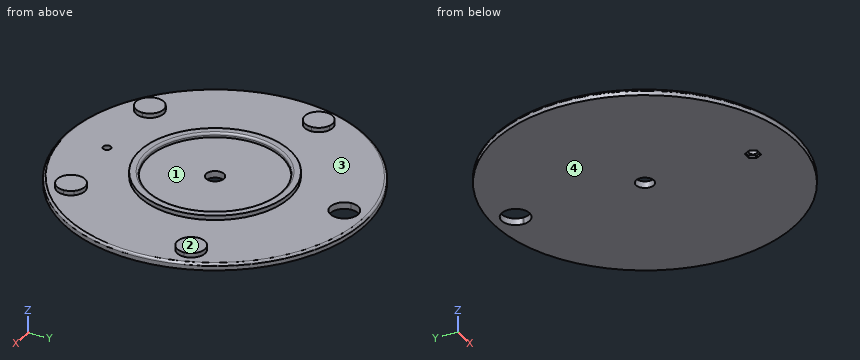
```python
from build123d import *

# Parameters (mm, degrees)
F0_R     = 67.5
F0_R_2   = 33.75
F1_DEPTH = 3
F0_R_3   = 30
F0_R_4   = 4
F2_DEPTH = 5
F3_START = 1
F0_R_5   = 1.75
F3_DEPTH = 2
F4_R     = 1


with BuildPart() as f1:
    # F0 (on Top) → F1 (new body)
    with BuildSketch(Plane.XY):
        Circle(F0_R)
        with BuildLine():
            ThreePointArc((-6.240649333, 56.8082458443), (-0.1709410263, 63.3976618959), (6.25, 57.15))
            ThreePointArc((6.25, 57.15), (6.2476618959, 56.9790589737), (6.240649333, 56.8082458443))
            ThreePointArc((6.240649333, 56.8082458443), (33.5919271685, 46.2353212285), (52.0993856897, 23.4899236005))
            ThreePointArc((52.0993856897, 23.4899236005), (57.8868692347, 22.8152624917), (60.6028799063, 17.6603212285))
            ThreePointArc((60.6028799063, 17.6603212285), (59.3068679409, 13.8497435095), (55.9563190893, 11.6195031725))
            ThreePointArc((55.9563190893, 11.6195031725), (56.8507965465, 5.8403280749), (57.15, 0))
            ThreePointArc((57.15, 0), (52.2635598843, -23.1223443496), (38.4398404822, -42.290674666))
            ThreePointArc((38.4398404822, -42.290674666), (39.480983044, -44.1421129506), (39.8419271685, -46.2353212285))
            ThreePointArc((39.8419271685, -46.2353212285), (35.3599862925, -52.2300244684), (28.3422577496, -49.6269979513))
            ThreePointArc((28.3422577496, -49.6269979513), (0, -57.15), (-28.3422577496, -49.6269979513))
            ThreePointArc((-28.3422577496, -49.6269979513), (-37.2655849953, -51.2916774434), (-38.4398404822, -42.290674666))
            ThreePointArc((-38.4398404822, -42.290674666), (-54.3528799063, -17.6603212285), (-55.9563190893, 11.6195031725))
            ThreePointArc((-55.9563190893, 11.6195031725), (-60.2969831331, 19.5916774434), (-52.0993856897, 23.4899236005))
            ThreePointArc((-52.0993856897, 23.4899236005), (-33.5919271685, 46.2353212285), (-6.240649333, 56.8082458443))
        make_face(mode=Mode.SUBTRACT)
        with BuildLine():
            ThreePointArc((6.240649333, 56.8082458443), (0, 50.9), (-6.240649333, 56.8082458443))
            ThreePointArc((-6.240649333, 56.8082458443), (-33.5919271685, 46.2353212285), (-52.0993856897, 23.4899236005))
            ThreePointArc((-52.0993856897, 23.4899236005), (-49.1979386431, 21.1943105569), (-48.1028799063, 17.6603212285))
            ThreePointArc((-48.1028799063, 17.6603212285), (-50.5423021872, 12.7063331939), (-55.9563190893, 11.6195031725))
            ThreePointArc((-55.9563190893, 11.6195031725), (-54.3528799063, -17.6603212285), (-38.4398404822, -42.290674666))
            ThreePointArc((-38.4398404822, -42.290674666), (-31.4987188906, -40.346265353), (-27.3419271685, -46.2353212285))
            ThreePointArc((-27.3419271685, -46.2353212285), (-27.5972239286, -48.0033803525), (-28.3422577496, -49.6269979513))
            ThreePointArc((-28.3422577496, -49.6269979513), (0, -57.15), (28.3422577496, -49.6269979513))
            ThreePointArc((28.3422577496, -49.6269979513), (29.9182693417, -41.1789650137), (38.4398404822, -42.290674666))
            ThreePointArc((38.4398404822, -42.290674666), (52.2635598843, -23.1223443496), (57.15, 0))
            ThreePointArc((57.15, 0), (56.8507965465, 5.8403280749), (55.9563190893, 11.6195031725))
            ThreePointArc((55.9563190893, 11.6195031725), (48.4087766794, 15.7289650137), (52.0993856897, 23.4899236005))
            ThreePointArc((52.0993856897, 23.4899236005), (33.5919271685, 46.2353212285), (6.240649333, 56.8082458443))
        make_face()
        Polygon((3.2331615075, -47.75), (1.6165807537, -50.55), (-1.6165807537, -50.55), (-3.2331615075, -47.75), (-1.6165807537, -44.95), (1.6165807537, -44.95), align=None, mode=Mode.SUBTRACT)
        Circle(F0_R_2, mode=Mode.SUBTRACT)
    extrude(amount=F1_DEPTH)



with BuildPart() as f1b:
    # F0 (on Top) → F1, piece 2 (new body)
    with BuildSketch(Plane.XY):
        Circle(F0_R_3)
        Circle(F0_R_4, mode=Mode.SUBTRACT)
    extrude(amount=F1_DEPTH)


with BuildPart() as f1_1:
    add(f1.part)

    add(f1b.part)  # F2 merges F1b
    # F0 (on Top) → F2 (join)
    with BuildSketch(Plane.XY):
        Circle(F0_R_2)
        Circle(F0_R_3, mode=Mode.SUBTRACT)
        with BuildLine():
            ThreePointArc((-48.1028799063, 17.6603212285), (-49.1979386431, 21.1943105569), (-52.0993856897, 23.4899236005))
            ThreePointArc((-52.0993856897, 23.4899236005), (-54.3528799063, 17.6603212285), (-55.9563190893, 11.6195031725))
            ThreePointArc((-55.9563190893, 11.6195031725), (-50.5423021872, 12.7063331939), (-48.1028799063, 17.6603212285))
        make_face()
        with BuildLine():
            ThreePointArc((-55.9563190893, 11.6195031725), (-54.3528799063, 17.6603212285), (-52.0993856897, 23.4899236005))
            ThreePointArc((-52.0993856897, 23.4899236005), (-60.2969831331, 19.5916774434), (-55.9563190893, 11.6195031725))
        make_face()
        with BuildLine():
            ThreePointArc((60.6028799063, 17.6603212285), (57.8868692347, 22.8152624917), (52.0993856897, 23.4899236005))
            ThreePointArc((52.0993856897, 23.4899236005), (54.3528799063, 17.6603212285), (55.9563190893, 11.6195031725))
            ThreePointArc((55.9563190893, 11.6195031725), (59.3068679409, 13.8497435095), (60.6028799063, 17.6603212285))
        make_face()
        with BuildLine():
            ThreePointArc((55.9563190893, 11.6195031725), (54.3528799063, 17.6603212285), (52.0993856897, 23.4899236005))
            ThreePointArc((52.0993856897, 23.4899236005), (48.4087766794, 15.7289650137), (55.9563190893, 11.6195031725))
        make_face()
        with BuildLine():
            ThreePointArc((28.3422577496, -49.6269979513), (33.5919271685, -46.2353212285), (38.4398404822, -42.290674666))
            ThreePointArc((38.4398404822, -42.290674666), (29.9182693417, -41.1789650137), (28.3422577496, -49.6269979513))
        make_face()
        with BuildLine():
            ThreePointArc((39.8419271685, -46.2353212285), (39.480983044, -44.1421129506), (38.4398404822, -42.290674666))
            ThreePointArc((38.4398404822, -42.290674666), (33.5919271685, -46.2353212285), (28.3422577496, -49.6269979513))
            ThreePointArc((28.3422577496, -49.6269979513), (35.3599862925, -52.2300244684), (39.8419271685, -46.2353212285))
        make_face()
        with BuildLine():
            ThreePointArc((-27.3419271685, -46.2353212285), (-31.4987188906, -40.346265353), (-38.4398404822, -42.290674666))
            ThreePointArc((-38.4398404822, -42.290674666), (-33.5919271685, -46.2353212285), (-28.3422577496, -49.6269979513))
            ThreePointArc((-28.3422577496, -49.6269979513), (-27.5972239286, -48.0033803525), (-27.3419271685, -46.2353212285))
        make_face()
        with BuildLine():
            ThreePointArc((-28.3422577496, -49.6269979513), (-33.5919271685, -46.2353212285), (-38.4398404822, -42.290674666))
            ThreePointArc((-38.4398404822, -42.290674666), (-37.2655849953, -51.2916774434), (-28.3422577496, -49.6269979513))
        make_face()
    extrude(amount=F2_DEPTH)

    # F0 (on Top) → F3 (join)
    with BuildSketch(Plane.XY.offset(F3_START)):
        Polygon((-1.6165807537, -50.55), (1.6165807537, -50.55), (3.2331615075, -47.75), (1.6165807537, -44.95), (-1.6165807537, -44.95), (-3.2331615075, -47.75), align=None)
        with Locations((0, -47.75)):
            Circle(F0_R_5, mode=Mode.SUBTRACT)
    extrude(amount=F3_DEPTH)

    # F4
    f4_edges = [f1_1.edges().sort_by_distance(p)[0] for p in [
        (-67.5, 0, 3),
        (-30, 0, 5),
    ]]
    fillet(f4_edges, radius=F4_R)


solid = f1_1.part
```
Verification items for the finished model (mm, model axes). Face numbers are marked on the shaded views. A direction names the side the tool comes from. Round coordinates to 2 decimals unless told otherwise and drop trailing zeros. Write each loop counter-clockwise with the first axis right and the second up, starting at its lowest first coordinate (ties: lowest second). Pieces come first, ordered by that corner, then holes.
1. Draft check along X on the marked faces 1 and 2. Enter one of: +X half, -X half, draft (parallel to the pull), parting line (faces both ways), or undercut.
2. Access from +Z, -Z, +X, -X, +Y, -Y to the whole of each face (thin tool, end or side, straight path). Record for the marked faces 3 and 4.
3. Gauge pin test, flat ends, axial feed: P1, Ø1, axis at x = -23.5, y = -45.5, coming from the +Z side; P2, Ø2, axis at y = 21.5, z = 4.5, coming from the -X side; P3, Ø5.5, axis at x = 0, y = -47.75, coming from the -Z side. Record the tip position at first contact, or that the pin passes through.
4. Section check B-B on y = 0. Enter the section's corners in (x, z).
5. Scan lines: L1, parallel to Y at x = 0, z = 1.45; L2, parallel to Y at x = 0, z = 3.5; L3, parallel to X at y = 15, z = 4. Record each from-to range of solid material in increasing order.
6. Section check A-A on x = 0. State how many separate pieces and enclosed holes the cut face has, plus the area to 3 significant figures.
Answer:
1. face 1: undercut
1. face 2: draft
2. face 3: +Z
2. face 4: -Z, +X, -X, +Y, -Y
3. P1: stops at z = 3
3. P2: stops at x = -59.92
3. P3: stops at z = 1
4. outline: (-67.5, 0) - (-4, 0) - (-4, 3) - (-30, 3) - (-30, 4) arc R1 ccw to (-31, 5) - (-33.75, 5) - (-33.75, 3) - (-66.5, 3) arc R1 ccw to (-67.5, 2) - close; (4, 0) - (67.5, 0) - (67.5, 2) arc R1 ccw to (66.5, 3) - (33.75, 3) - (33.75, 5) - (31, 5) arc R1 ccw to (30, 4) - (30, 3) - (4, 3) - close
5. L1: y = -67.5 to -49.5, -46 to -4, 4 to 50.9, 63.4 to 67.5
5. L2: y = -33.75 to -30, 30 to 33.75
5. L3: x = -60.01 to -48.7, -30.23 to -25.98, 25.98 to 30.23, 48.7 to 60.01
6. separate pieces: 4
6. enclosed holes: 0
6. area: 345 mm2
